from build123d import *

# Parameters (mm, degrees)
SKETCH_1_R          = 2.025
SKETCH_1_R_2        = 13.1
SKETCH_1_R_3        = 3
EXTRUDE_1_DEPTH     = 5
CUT_EXTRUDE_3_DEPTH = 10
FILLET_2_R          = 3
SKETCH_5_R          = 1.525
CUT_EXTRUDE_4_DEPTH = 20


with BuildPart() as part:
    # 草图1 → 凸台-拉伸1 (new body)
    with BuildSketch(Plane(origin=(0, 0, 0), x_dir=(1, 0, 0), z_dir=(0, 1, 0))):
        with BuildLine():
            Line((76.972140647, 43.13107423), (-4.193547259, 32.732463418))
            ThreePointArc((-4.193547259, 32.732463418), (-32.337515252, -6.579141836), (8.929411765, -31.768940894))
            Line((8.929411765, -31.768940894), (87.705882353, -9.626951786))
            ThreePointArc((87.705882353, -9.626951786), (94.014523475, -4.328783491), (94.205048973, 3.907310252))
            ThreePointArc((94.205048973, 3.907310252), (89.748559809, 18.25955029), (88.242912543, 33.212145922))
            ThreePointArc((88.242912543, 33.212145922), (84.849435117, 40.719066694), (76.972140647, 43.13107423))
        make_face()
        with Locations((0, 17.5)):
            Circle(SKETCH_1_R, mode=Mode.SUBTRACT)
        with Locations((8.75, 15.155444566)):
            Circle(SKETCH_1_R, mode=Mode.SUBTRACT)
        with Locations((-8.75, -15.155444566)):
            Circle(SKETCH_1_R, mode=Mode.SUBTRACT)
        with Locations((0, -17.5)):
            Circle(SKETCH_1_R, mode=Mode.SUBTRACT)
        with Locations((-15.155444566, -8.75)):
            Circle(SKETCH_1_R, mode=Mode.SUBTRACT)
        with Locations((8.75, -15.155444566)):
            Circle(SKETCH_1_R, mode=Mode.SUBTRACT)
        with Locations((15.155444566, -8.75)):
            Circle(SKETCH_1_R, mode=Mode.SUBTRACT)
        with Locations((-17.5, 0)):
            Circle(SKETCH_1_R, mode=Mode.SUBTRACT)
        Circle(SKETCH_1_R_2, mode=Mode.SUBTRACT)
        with Locations((-15.155444566, 8.75)):
            Circle(SKETCH_1_R, mode=Mode.SUBTRACT)
        with Locations((17.5, 0)):
            Circle(SKETCH_1_R, mode=Mode.SUBTRACT)
        with Locations((15.155444566, 8.75)):
            Circle(SKETCH_1_R, mode=Mode.SUBTRACT)
        with Locations((-8.75, 15.155444566)):
            Circle(SKETCH_1_R, mode=Mode.SUBTRACT)
        with Locations((85, 0)):
            Circle(SKETCH_1_R_3, mode=Mode.SUBTRACT)
        with Locations((78.242912543, 33.212145922)):
            Circle(SKETCH_1_R_3, mode=Mode.SUBTRACT)
    extrude(amount=EXTRUDE_1_DEPTH)

    # 草图4 → 切除-拉伸3 (cut)
    with BuildSketch(Plane.XZ):
        with BuildLine():
            Line((76.108728609, 4.576602785), (25.994527014, 18.662383699))
            ThreePointArc((25.994527014, 18.662383699), (30.461655113, 9.802426627), (32, 0))
            ThreePointArc((32, 0), (31.185942012, -7.171960739), (28.785186198, -13.979021981))
            Line((28.785186198, -13.979021981), (76.108728609, 4.576602785))
        make_face()
        Polygon((69.770383541, -34.143027562), (16.636114037, -27.335685646), (75.881597407, -4.105451761), align=None)
    extrude(amount=-CUT_EXTRUDE_3_DEPTH, mode=Mode.SUBTRACT)

    # 圆角2
    fillet_2_edges = [part.edges().sort_by_distance(p)[0] for p in [
        (69.770383541, 2.5, -34.143027562),
        (16.636114037, 2.5, -27.335685646),
        (75.881597407, 2.5, -4.105451761),
        (28.785186198, 2.5, -13.979021981),
        (25.994527014, 2.5, 18.662383699),
        (76.108728609, 2.5, 4.576602785),
    ]]
    fillet(fillet_2_edges, radius=FILLET_2_R)

    # 草图5 → 切除-拉伸4 (cut)
    with BuildSketch(Plane(origin=(0, 5, 0), x_dir=(1, 0, 0), z_dir=(0, 1, 0))):
        with Locations((-27.522163408, 0)):
            Circle(SKETCH_5_R)
        with Locations((0, 27.522163408)):
            Circle(SKETCH_5_R)
        with Locations((0, -27.522163408)):
            Circle(SKETCH_5_R)
        with Locations((30.901702525, -21.438107622)):
            Circle(SKETCH_5_R)
        with Locations((54.969081991, -14.673401739)):
            Circle(SKETCH_5_R)
        with Locations((33.321534862, 16.496811603)):
            Circle(SKETCH_5_R)
        with Locations((56.596303964, 7.370743267)):
            Circle(SKETCH_5_R)
    extrude(amount=-CUT_EXTRUDE_4_DEPTH, mode=Mode.SUBTRACT)


solid = part.part
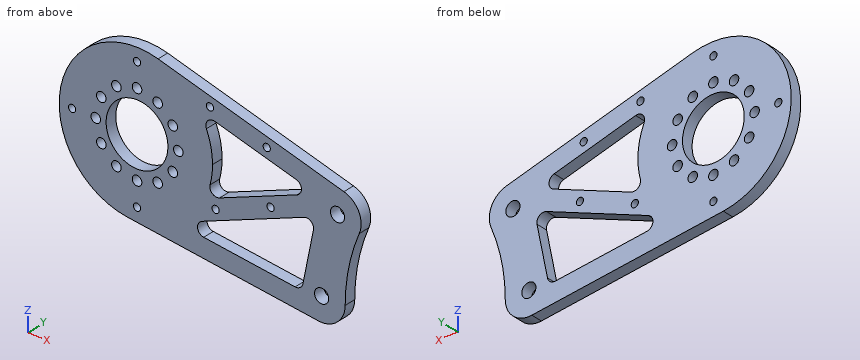
Verification items for the finished model (mm, model axes). Coordinates: 2 decimals unless noted, no trailing zeros. Loops run counter-clockwise (first coordinate to the right, second up) from the corner with the lowest first, then second, coordinate; pieces in that order, holes last. Notation, with made-up numbers: (18, 82) -> (60, 82) arc R10 ccw to (60, 89) -> close; hole circle Ø5 at (56, 7). An arc over 180 degrees is marked (long way). Answer as a JSON object with one key per item and string values. Group by question number.
Item 1: Scan lines: probe 1 along Z at (x, y) = (68, 4.3); probe 2 along Z at (x, y) = (0, 1.3) (3 decimals); probe 3 along Z at (x, y) = (66.5, 2.45). Record each from-to range of solid material in increasing order.
Item 2: Sectioned sample at A-A on x = 85. Record the boundary of the cut face in (y, z).
Item 3: Sectioned sample at B-B on y = 1.6. State how many separate pieces and enclosed holes the cut face has, plus the area to 3 significant figures.
Item 4: Depth check by flat-ended pin: pin 1 (2.5 mm diameter, centred on x = 56.6, z = -7.37, fed in from -Y); pin 2 (3 mm diameter, centred on x = 77, y = 4, fed in from +Z). Enter the tip coordinate at first touch or a pass-through.
Evaluation:
{
 "1": {"probe 1": "z = -41.98 to -33.75, -7.2 to 1.41, 6.81 to 15.17", "probe 2": "z = -33.27 to -29.047, -25.997 to -19.525, -15.475 to -13.1, 13.1 to 15.475, 19.525 to 25.997, 29.047 to 33", "probe 3": "z = -41.79 to -33.72, -7.78 to 0.81, 7.28 to 15.59"},
 "2": {"outline": "(0, -40.58) -> (5, -40.58) -> (5, -3) -> (0, -3) -> close; (0, 3) -> (5, 3) -> (5, 10.39) -> (0, 10.39) -> close"},
 "3": {"separate pieces": "1", "enclosed holes": "24", "area": "4,920 mm²"},
 "4": {"pin 1": "passes through", "pin 2": "stops at z = 13.06"}
}
